Autodesk Inventor part; units mm, degrees
ref_plane "YZ Plane" through (0, 0, 0) normal (1, 0, 0) x (0, 1, 0)
ref_plane "XZ Plane" through (0, 0, 0) normal (0, 1, 0) x (-1, 0, 0)
ref_plane "XY Plane" through (0, 0, 0) normal (0, 0, 1) x (1, 0, 0)
sketch "Эскиз1" plane through (0, 0, 0) normal (0, 0, 1) x (1, 0, 0)
  line L0 (-8.4853, 57.9828) -> (-57.9828, 8.4853)
  line L1 (-57.9828, -8.4853) -> (-8.4853, -57.9828)
  line L2 (8.4853, -57.9828) -> (57.9828, -8.4853)
  line L3 (57.9828, 8.4853) -> (8.4853, 57.9828)
  line L4 (-93.0553, 0) -> (93.0553, 0)
  line L5 (0, -87.0906) -> (0, 92.0611)
  arc A0 (-57.9828, 8.4853) -> (-57.9828, -8.4853) centre (-49.4975, 0) ccw
  arc A1 (8.4853, 57.9828) -> (-8.4853, 57.9828) centre (0, 49.4975) ccw
  arc A2 (57.9828, -8.4853) -> (57.9828, 8.4853) centre (49.4975, 0) ccw
  arc A3 (-8.4853, -57.9828) -> (8.4853, -57.9828) centre (0, -49.4975) ccw
  point P0 (0, 66.468)
  point P1 (-66.468, 0)
  point P2 (66.468, 0)
  dimension "d5" = 94
  dimension "d7" = 94
  dimension "d8" = 12
extrude "Выдавливание1" add sketch "Эскиз1" along normal blind 40
sketch "Эскиз2" plane through (0, 0, 40) normal (0, 0, 1) x (1, 0, 0)
  circle A0 centre (0, 0) radius 54
  dimension "d11" = 108
extrude "Выдавливание2" add sketch "Эскиз2" along normal blind 88
sketch "Эскиз3" plane through (0, 0, 128) normal (0, 0, 1) x (1, 0, 0)
  circle A0 centre (0, 0) radius 42
  dimension "d14" = 84
extrude "Выдавливание3" cut sketch "Эскиз3" against normal blind 79
sketch "Эскиз4" plane through (0, 0, 0) normal (0, 0, -1) x (-1, 0, 0)
  circle A0 centre (0, 0) radius 36
  dimension "d17" = 72
extrude "Выдавливание4" cut sketch "Эскиз4" against normal blind 40
chamfer "Фаска1" distance 2 angle 45 1 edges at (-54, 0, 128)
chamfer "Фаска2" distance 1.6 angle 45 1 edges at (36, 0, 0)
sketch "Эскиз6" plane through (0, 0, 0) normal (0, 0, -1) x (-1, 0, 0)
  circle A0 centre (0, 49) radius 6
  circle A1 centre (0, -49) radius 6
  line L0 (86.0965, 0) -> (-86.0965, 0)
  circle A2 centre (49, 0) radius 6
  circle A3 centre (-49, 0) radius 6
  line L1 (0, -86.0965) -> (0, 86.0965)
  point P0 (0, 0)
  dimension "d30" = 98
  dimension "d31" = 12
  dimension "d32" = 12
  dimension "d33" = 98
  dimension "d34" = 12
  dimension "d35" = 12
fillet "Сопряжение1" radius 2 5 edges at (0, 54, 40) (-54, 0, 40) (0, -54, 40) (53.5066, -7.2827, 40) (53.5066, 7.2827, 40)
hole "Отверстие1" at (49, 0, 0) direction (0, 0, 1) diameter 10.106 depth 30.5 tip angle 118
chamfer "Фаска3" distance 2 angle 45 1 edges at (49, -5.053, 0)
sketch "Эскиз7" plane through (0, 0, 0) normal (0, 0, -1) x (-1, 0, 0)
  circle A0 centre (49, 0) radius 6
  point P0 (0, 0)
  dimension "d47" = 49
  dimension "d48" = 12
hole "Отверстие2" at (-49, 0, 0) direction (0, 0, 1) diameter 10.106 depth 30.5 tip angle 118
chamfer "Фаска4" distance 2 angle 45 1 edges at (-49, -5.053, 0)
sketch "Эскиз8" plane through (0, 0, 0) normal (0, 0, -1) x (-1, 0, 0)
  circle A0 centre (0, 49) radius 6
  point P0 (0, 0)
  dimension "d59" = 12
  dimension "d60" = 49
hole "Отверстие3" at (0, 49, 0) direction (0, 0, 1) diameter 10.106 depth 30.5 tip angle 118
chamfer "Фаска5" distance 2 angle 45 1 edges at (0, 43.947, 0)
sketch "Эскиз9" plane through (0, 0, 0) normal (0, 0, -1) x (-1, 0, 0)
  circle A0 centre (0, -49) radius 6
  point P0 (0, 0)
  dimension "d71" = 12
  dimension "d72" = 49
hole "Отверстие4" at (0, -49, 0) direction (0, 0, 1) diameter 10.106 depth 30.5 tip angle 118
chamfer "Фаска6" distance 2 angle 45 1 edges at (0, -54.053, 0)
properties part number "Пункт 1(чё там считать)"
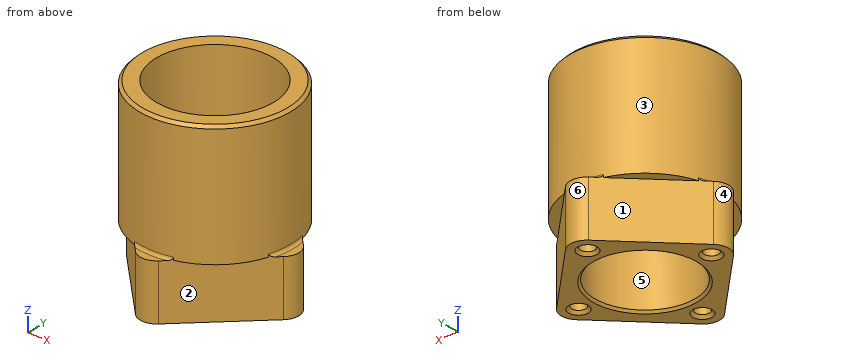
Check sheet for the modelled part. Datum: model origin and axes. Units: mm. Face numbers are marked on the shaded views. A direction names the side the tool comes from. Round coordinates to 2 decimals unless told otherwise and drop trailing zeros. Loops run counter-clockwise (first coordinate to the right, second up) from the corner with the lowest first, then second, coordinate; pieces in that order, holes last. Notation, with made-up numbers: M -17.5,-13.5 L -9.5,-13.5 A6 ccw -9.5,-8.5 Z; hole C 77,-4.75 d7. An arc over 180 degrees is marked long. One line per item, written item: value.
(1) Depth check by flat-ended pin: pin 1 Ø3.5 at (x, y) = (3, 59) entering from +Z; pin 2 Ø12 at (y, z) = (-40.5, 50.5) entering from -X; pin 3 Ø10 at (x, z) = (19.5, 42) entering from -Y. Enter the tip coordinate at first touch or a pass-through.
Computed values:
pin 1: stops at z = 40
pin 2: stops at x = -41.54
pin 3: stops at y = -52.02
(2) Sectioned sample at A-A, the plane z = 23. Record the cut outline in (x, y).
Computed values:
outline: M -57.98,-8.49 L -8.49,-57.98 A12 ccw 8.49,-57.98 L 57.98,-8.49 A12 ccw 57.98,8.49 L 8.49,57.98 A12 ccw -8.49,57.98 L -57.98,8.49 A12 ccw Z; hole C -49,0 d10.11; hole C 0,0 d72; hole C 0,-49 d10.11; hole C 0,49 d10.11; hole C 49,0 d10.11
(3) Thickness scan on line 1 (Y direction, x = 0, z = 19); line 2 (Y direction, x = 0, z = 111); line 3 (X direction, y = -1.5, z = 18.5). Record the ranges inside material, lowest first.
Computed values:
line 1: y = -61.5 to -54.05, -43.95 to -36, 36 to 43.95, 54.05 to 61.5
line 2: y = -54 to -42, 42 to 54
line 3: x = -61.4 to -53.83, -44.17 to -35.97, 35.97 to 44.17, 53.83 to 61.4
(4) Release check for a two-part mould opening along X. For the marked faces 4, 5 and 6 record: +X half, -X half, draft (parallel to the pull), parting line (faces both ways), or undercut.
Computed values:
face 4: -X half
face 5: undercut
face 6: parting line
(5) Sectioned sample at B-B, the plane z = 79. Record the cut outline in (x, y), then the cut area to 3 significant figures.
Computed values:
outline: C 0,0 d108; hole C 0,0 d84
area: 3,620 mm^2
(6) Access from +Z, -Z, +X, -X, +Y, -Y to the whole of each face (thin tool, end or side, straight path). Record for the marked faces 1, 2 and 3.
Computed values:
face 1: -Z, -X, +Y
face 2: -Z, +X, -Y
face 3: +Z
